Read the model definition and answer for the solid it produces. Units are mm, in the model's axes. Face numbers are marked on the shaded views. A direction names the side the tool comes from. Coordinates: 2 decimals unless noted, no trailing zeros. Loops run counter-clockwise (first coordinate to the right, second up) from the corner with the lowest first, then second, coordinate; pieces in that order, holes last. Notation, with made-up numbers: M 30.25,-24.5 L 49.25,-24.5 A13 cw 49.25,-2.5 Z; hole C 26.5,32 d9. An arc over 180 degrees is marked long. One line per item, written item: value. Start each with the question number.
1. Flat-ended cylindrical pins translate along their axes: pin 1 (2 mm diameter, centred on x = 4.5, z = 24.5, fed in from -Y); pin 2 (1.5 mm diameter, centred on x = -4, y = 38, fed in from +Z); pin 3 (0.6 mm diameter, centred on x = 1, z = 1, fed in from -Y). Find the tip coordinate at first contact, or state that the pin passes through.
2. The part is cut by section C-C (z = 23). Write down the section's boundary in (x, y).
3. Consider probe 1 along X at (y, z) = (0, 1.4); probe 2 along Z at (x, y) = (-1.25, 17.5); probe 3 along Y at (x, z) = (-0.75, 11). Determine where each line is inside the solid, lowest interval first.
4. For the marked faces 1 and 2, determine the directions among +Z, -Z, +X, -X, +Y, -Y from which every point of the face is accessible in a straight line to the end or side of a thin tool.
5. The part is cut by section B-B (y = 6). Write down the section's boundary in (x, z), then the cut area to 3 significant figures.
6. The part is cut by section A-A (x = -1.25). Write down the section's boundary in (y, z).
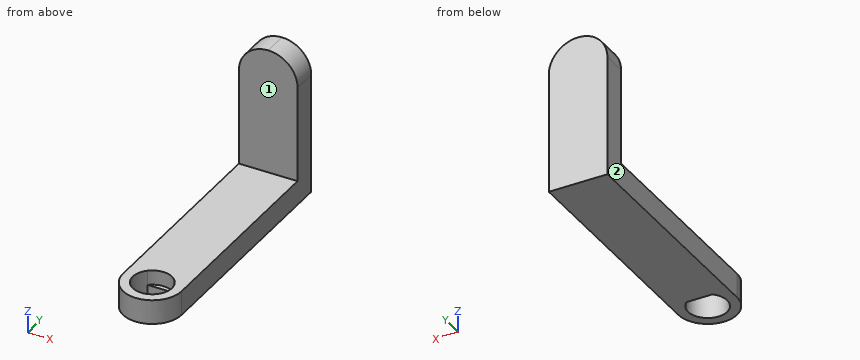
```python
from build123d import *
from build123d.topology import SkipClean

# Parameters (mm, degrees)
SKETCH1_R           = 6
BOSS_EXTRUDE1_DEPTH = 5
BOSS_EXTRUDE2_START = -5
BOSS_EXTRUDE2_DEPTH = 5
CUT_EXTRUDE1_START  = -3
SKETCH3_R           = 4
CUT_EXTRUDE1_DEPTH  = 3
SKETCH4_W           = 12
SKETCH4_H           = 5
BOSS_EXTRUDE3_DEPTH = 25.73
FILLET1_R           = 6


with BuildPart() as part:
    # Sketch1 → Boss-Extrude1 (new body)
    with BuildSketch(Plane.XY):
        Circle(SKETCH1_R)
        with BuildLine():
            Line((-2.645751311, 3), (2.645751311, 3))
            ThreePointArc((2.645751311, 3), (0, -4), (-2.645751311, 3))
        make_face(mode=Mode.SUBTRACT)
    extrude(amount=BOSS_EXTRUDE1_DEPTH)

    # Sketch2 → Boss-Extrude2 (add)
    with BuildSketch(Plane.XY.offset(5).offset(BOSS_EXTRUDE2_START)):
        with BuildLine():
            Line((-6, 0), (-6, 47.2))
            Line((-6, 47.2), (6, 47.2))
            Line((6, 47.2), (6, 0))
            ThreePointArc((6, 0), (0, 6), (-6, 0))
        make_face()
    extrude(amount=BOSS_EXTRUDE2_DEPTH)

    # Sketch3 → Cut-Extrude1 (cut)
    with SkipClean():  # the faces are left unmerged after this step: merging them gives an invalid solid
        with BuildSketch(Plane.XY.offset(5).offset(CUT_EXTRUDE1_START)):
            with Locations(Location((0, 0, 0), (0, 0, 131.409622109))):
                Circle(SKETCH3_R)
        extrude(amount=CUT_EXTRUDE1_DEPTH, mode=Mode.SUBTRACT)

    # Sketch4 → Boss-Extrude3 (add)
    with SkipClean():  # the faces are left unmerged after this step: merging them gives an invalid solid
        with BuildSketch(Plane.XY.offset(5)):
            with Locations((0, 44.7)):
                Rectangle(SKETCH4_W, SKETCH4_H)
        extrude(amount=BOSS_EXTRUDE3_DEPTH)

    # Fillet1
    fillet1_edges = [part.edges().sort_by_distance(p)[0] for p in [
        (-6, 44.7, 30.73),
        (6, 44.7, 30.73),
    ]]
    fillet(fillet1_edges, radius=FILLET1_R - 0.0001)  # a hair under: the kernel refuses the full size


solid = part.part
```
Answer block:
1. pin 1: stops at y = 42.2
1. pin 2: stops at z = 5
1. pin 3: stops at y = -5.96
2. outline: M -6,42.2 L 6,42.2 L 6,47.2 L -6,47.2 Z
3. probe 1: x = -6 to -4, 4 to 6
3. probe 2: z = 0 to 5
3. probe 3: y = 42.2 to 47.2
4. face 1: +Z, +X, -X, -Y
4. face 2: +Z, -Z, -X, +Y, -Y
5. outline: M -6,0 L 6,0 L 6,5 L -6,5 Z
5. area: 60.0 mm2
6. outline: M -5.87,0 L -3.8,0 L -3.8,5 L -5.87,5 Z; M 3,0 L 47.2,0 L 47.2,30.6 L 42.2,30.6 L 42.2,5 L 3.8,5 L 3.8,2 L 3,2 Z
